```python
from build123d import *

# Parameters (mm, degrees)
SKETCH1_R           = 25
BOSS_EXTRUDE1_DEPTH = 10


with BuildPart() as part:
    # Sketch1 → Boss-Extrude1 (new body, symmetric)
    with BuildSketch(Plane.XY):
        with BuildLine():
            Line((-2300, 110.00001646), (-2309.84807753, 111.736498237))
            Line((-2309.84807753, 111.736498237), (-2344.209578927, -83.137259929))
            Line((-2344.209578927, -83.137259929), (-2349.419024257, -112.681492519))
            Line((-2349.419024257, -112.681492519), (-2144.255152103, -148.857418644))
            Line((-2144.255152103, -148.857418644), (-2137.403540795, -110))
            Line((-2137.403540795, -110), (0, -110))
            ThreePointArc((0, -110), (110.00000823, 8.23e-06), (0, 110.00001646))
            Line((0, 110.00001646), (-2300, 110.00001646))
        make_face()
        with Locations((0, 8.23e-06)):
            Circle(SKETCH1_R, mode=Mode.SUBTRACT)
    extrude(amount=BOSS_EXTRUDE1_DEPTH, both=True)


solid = part.part
```
The listing builds one solid part. Answer for the finished solid, in the listing's coordinates (mm). Round coordinates to 2 decimals unless told otherwise and drop trailing zeros. Loops run counter-clockwise (first coordinate to the right, second up) from the corner with the lowest first, then second, coordinate; pieces in that order, holes last.
Q1. Section A-A, the plane z = 4 is taken. Determine the outline of the cut face in (x, y).
Q2. Given pin 1 Ø3 at (y, z) = (-89.5, -4) entering from +X; pin 2 Ø5 at (x, z) = (-995, -1.5) entering from +Y; pin 3 Ø1.5 at (y, z) = (-77.5, -2.5) entering from +X, each flat-ended and moving along its own axis, determine where each tip first touches the part or whether it passes through.
Q3. Section B-B, the plane x = -1587 is taken. Determine the outline of the cut face in (y, z), then the cut area to 3 significant figures.
Q4. Find the intervals of material crossed by line 1 (Y direction, x = -4.5, z = 5.5); line 2 (Y direction, x = -904, z = 6.5); line 3 (X direction, y = -2, z = -3), in increasing order.
Q5. For a pull along Y with two mould halves and no side action, classify faces 1 (the face through (-1137, -17, -10)), 2 (the face through (11.5, -22.2, -0.1)), 3 (the face through (-2329.357, 1.098, 0.14)) as released by +Y, released by -Y, zero draft, split by the parting line, or undercut.
Completed:
1. outline: (-2349.42, -112.68) - (-2144.26, -148.86) - (-2137.4, -110) - (0, -110) arc R110 ccw to (0, 110) - (-2300, 110) - (-2309.85, 111.74) - close; hole circle Ø50 at (0, 0)
2. pin 1: stops at x = 66
2. pin 2: stops at y = 110
2. pin 3: stops at x = 78.8
3. outline: (-110, -10) - (110, -10) - (110, 10) - (-110, 10) - close
3. area: 4,400 mm2
4. line 1: y = -110 to -24.59, 24.59 to 110
4. line 2: y = -110 to 110
4. line 3: x = -2329.9 to -24.92, 24.92 to 109.98
5. face 1: zero draft
5. face 2: undercut
5. face 3: released by +Y
